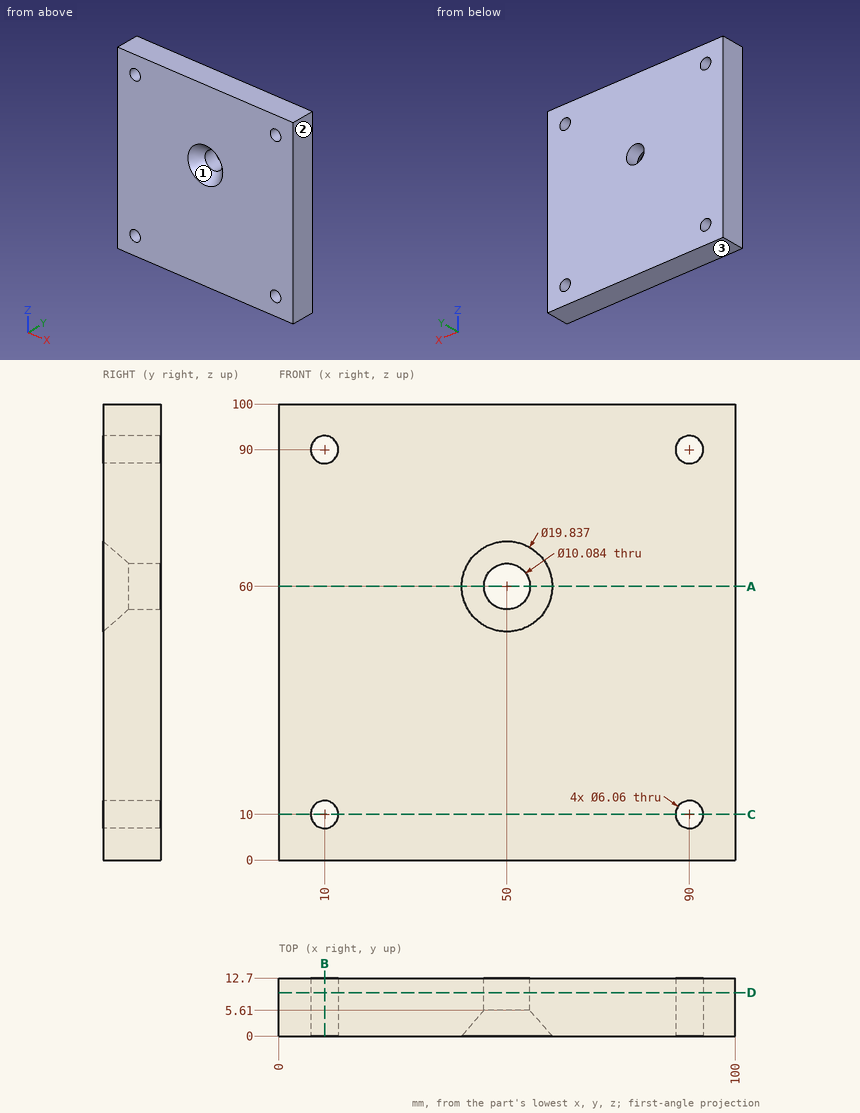
Geometry: see drawing. Coordinates: mm, zero at the bounding-box minimum. Give positions to 0.01 mm unless a question says otherwise; leave off trailing zeros. Order: outer loops, then holes, each group sorted by start corner. A loop starts at its lowest first (then second) coordinate and runs counter-clockwise, first axis right, second up.
Q1. Section D-D on y = 9.5. Output: boundary loops of the cut face in (x, z).
Checked values:
outline: (0, 0) - (100, 0) - (100, 100) - (0, 100) - close; hole circle Ø6.06 at (10, 10); hole circle Ø6.06 at (10, 90); hole circle Ø10.08 at (50, 60); hole circle Ø6.06 at (90, 10); hole circle Ø6.06 at (90, 90)
Q2. Draft query along Z for the marked faces 1, 2 and 3. Return one class per face: +Z half, -Z half, draft (parallel to the pull), parting line (faces both ways), or undercut.
Checked values:
face 1: undercut
face 2: draft
face 3: -Z half
Q3. Ray query, probe 1 along X at (y, z) = (3, 90); probe 2 along Z at (x, y) = (92, 11.75) (1 decimal). Return the intervals inside material, ascending.
Checked values:
probe 1: x = 0 to 6.97, 13.03 to 86.97, 93.03 to 100
probe 2: z = 0 to 7.7, 12.3 to 87.7, 92.3 to 100
Q4. Contact query for a flat-ended pin moving along its axis: pin 1 Ø1 at (x, z) = (51.5, 64.5) entering from -Y. Output: stop coordinate, or through.
Checked values:
pin 1: stops at y = 5.38
Q5. Section B-B on x = 10. Output: boundary loops of the cut face in (y, z), and give its area (3 significant figures).
Checked values:
outline: (0, 0) - (12.7, 0) - (12.7, 6.97) - (0, 6.97) - close; (0, 13.03) - (12.7, 13.03) - (12.7, 86.97) - (0, 86.97) - close; (0, 93.03) - (12.7, 93.03) - (12.7, 100) - (0, 100) - close
area: 1,120 mm2
Q6. Section A-A on z = 60. Output: boundary loops of the cut face in (x, y), and give its area (3 significant figures).
Checked values:
outline: (0, 0) - (40.08, 0) - (44.96, 5.61) - (44.96, 12.7) - (0, 12.7) - close; (55.04, 5.61) - (59.92, 0) - (100, 0) - (100, 12.7) - (55.04, 12.7) - close
area: 1,110 mm2
Q7. Section C-C on z = 10. Output: boundary loops of the cut face in (x, y), and give its area (3 significant figures).
Checked values:
outline: (0, 0) - (6.97, 0) - (6.97, 12.7) - (0, 12.7) - close; (13.03, 0) - (86.97, 0) - (86.97, 12.7) - (13.03, 12.7) - close; (93.03, 0) - (100, 0) - (100, 12.7) - (93.03, 12.7) - close
area: 1,120 mm2
